Job drawing, mm, ordinate dimensions from the low corner. One solid piece. Round coordinates to 2 decimals unless told otherwise and drop trailing zeros. Write each loop counter-clockwise with the first axis right and the second up, starting at its lowest first coordinate (ties: lowest second). Pieces come first, ordered by that corner, then holes. Notation, with made-up numbers: (5, 33) - (45, 33) arc R28 ccw to (45, 72) - close; hole circle Ø8 at (13, 49.5). An arc over 180 degrees is marked (long way). Write each question's results on one line, items separated by ' | '.
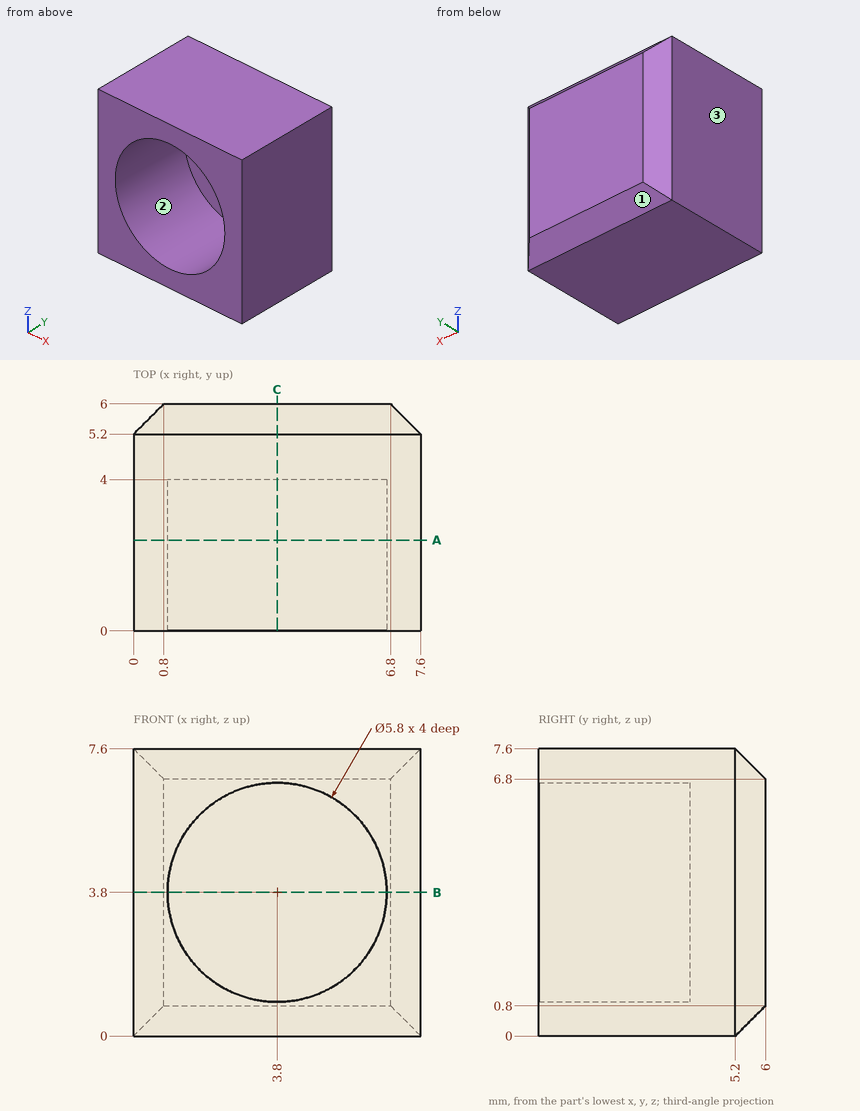
(1) Slice it at A-A, the plane y = 2.4. Write the cut outline in (x, z).
Worked answers:
outline: (0, 0) - (7.6, 0) - (7.6, 7.6) - (0, 7.6) - close; hole circle Ø5.8 at (3.8, 3.8)
(2) Drill centre lines: probe 1 along Z at (x, y) = (3.8, 1.8); probe 2 along Y at (x, z) = (4, 3); probe 3 along Z at (x, y) = (1.25, 2.3). Where is each one in solid material? Low to high. Write a range as [from, to].
Worked answers:
probe 1: z = [0, 0.9], [6.7, 7.6] | probe 2: y = [4, 6] | probe 3: z = [0, 2.42], [5.18, 7.6]
(3) Two-plate mould, pull along Z, no slides. Class the marked faces 1, 2 and 3: released by +Z, released by -Z, zero draft, split by the parting line, or undercut.
Worked answers:
face 1: released by -Z | face 2: undercut | face 3: zero draft
(4) Slice it at C-C, the plane x = 3.8. Write the cut outline in (y, z), and give its area (3 significant figures).
Worked answers:
outline: (0, 0) - (5.2, 0) - (6, 0.8) - (6, 6.8) - (5.2, 7.6) - (0, 7.6) - (0, 6.7) - (4, 6.7) - (4, 0.9) - (0, 0.9) - close | area: 21.8 mm2
(5) Slice it at B-B, the plane z = 3.8. Write the cut outline in (x, y), and give its area (3 significant figures).
Worked answers:
outline: (0, 0) - (0.9, 0) - (0.9, 4) - (6.7, 4) - (6.7, 0) - (7.6, 0) - (7.6, 5.2) - (6.8, 6) - (0.8, 6) - (0, 5.2) - close | area: 21.8 mm2
